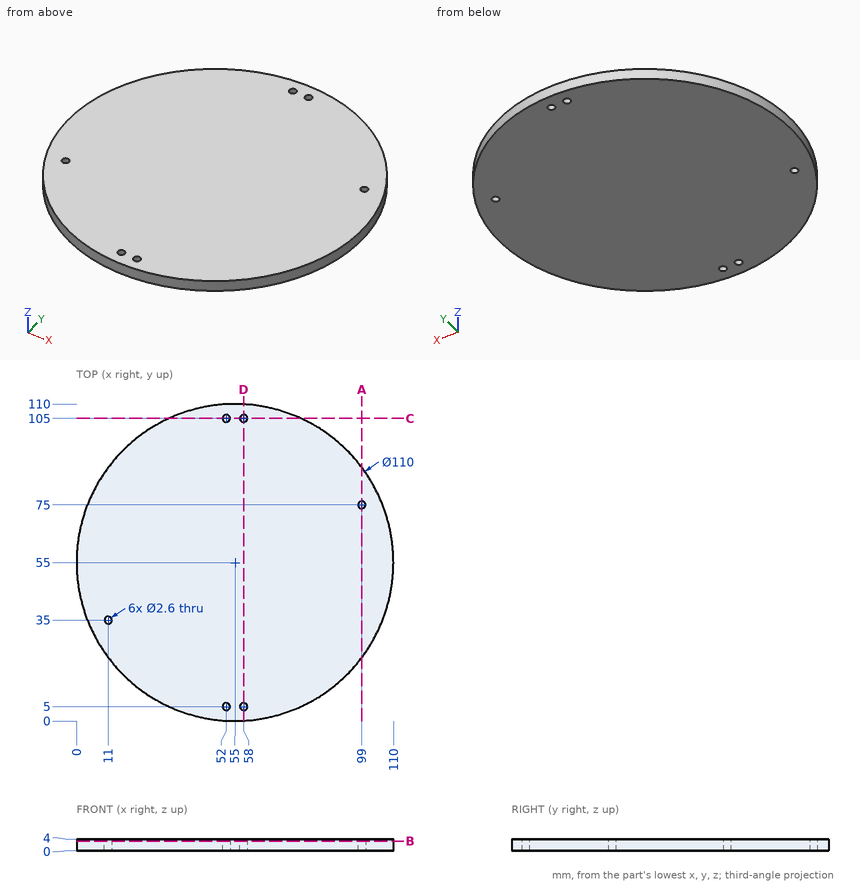
Study the drawing (mm; zero at the part's minimum x, y, z) and answer. Give positions to 0.01 mm unless a question says otherwise; leave off trailing zeros. Write each loop counter-clockwise with the first axis right and the second up, starting at its lowest first coordinate (ties: lowest second). Pieces come first, ordered by that corner, then holes. Notation, with made-up numbers: M 11.5,4.25 L 27.5,4.25 A30 cw 27.5,34.25 Z; hole C 65,-25 d3. An arc over 180 degrees is marked long. Put each result on its own line as item: value. Start each with the question number.
1. This flat-tipped pin is pushed along its axis until it touches: pin 1 Ø2 at (x, y) = (52, 105) entering from -Z. Where does it stop, or does it pass through?
2. The part is cut by section B-B, the plane z = 3.3. Give the vertices of the cut face in (x, y).
3. Consider line 1 along Y through (x, z) = (58, 2); line 2 along X through (y, z) = (105, 2.8); line 3 along Y through (x, z) = (11, 1.45). Determine where each line is inside the solid, lowest interval first.
4. The part is cut by section C-C, the plane y = 105. Give the vertices of the cut face in (x, z), and give its area (3 significant figures).
5. The part is cut by section A-A, the plane x = 99. Give the vertices of the cut face in (y, z).
6. The part is cut by section D-D, the plane x = 58. Give the vertices of the cut face in (y, z), and give its area (3 significant figures).
Final values:
1. pin 1: passes through
2. outline: C 55,55 d110; hole C 11,35 d2.6; hole C 52,5 d2.6; hole C 52,105 d2.6; hole C 58,5 d2.6; hole C 58,105 d2.6; hole C 99,75 d2.6
3. line 1: y = 0.08 to 3.7, 6.3 to 103.7, 106.3 to 109.92
3. line 2: x = 32.09 to 50.7, 53.3 to 56.7, 59.3 to 77.91
3. line 3: y = 22 to 33.7, 36.3 to 88
4. outline: M 32.09,0 L 50.7,0 L 50.7,4 L 32.09,4 Z; M 53.3,0 L 56.7,0 L 56.7,4 L 53.3,4 Z; M 59.3,0 L 77.91,0 L 77.91,4 L 59.3,4 Z
4. area: 163 mm²
5. outline: M 22,0 L 73.7,0 L 73.7,4 L 22,4 Z; M 76.3,0 L 88,0 L 88,4 L 76.3,4 Z
6. outline: M 0.08,0 L 3.7,0 L 3.7,4 L 0.08,4 Z; M 6.3,0 L 103.7,0 L 103.7,4 L 6.3,4 Z; M 106.3,0 L 109.92,0 L 109.92,4 L 106.3,4 Z
6. area: 419 mm²
